Geometry: final body of the model. Coordinates: model frame, mm. Face numbers are marked on the shaded views. A direction names the side the tool comes from. Coordinates: 2 decimals unless noted, no trailing zeros. Write each loop counter-clockwise with the first axis right and the second up, starting at its lowest first coordinate (ties: lowest second). Pieces come first, ordered by that corner, then holes. Notation, with made-up numbers: (9, 46.5) -> (67, 46.5) arc R28 ccw to (67, 78.5) -> close; hole circle Ø6 at (0, 77). An arc over 180 degrees is marked (long way). One line per item, written item: value.
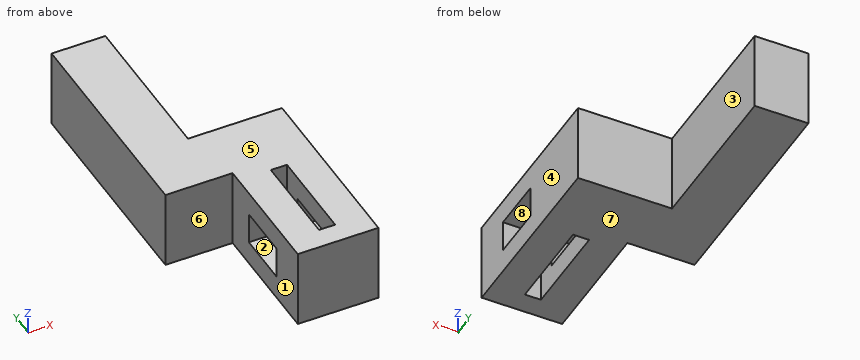
```python
from build123d import *

# Parameters (mm, degrees)
SKETCH1_W           = 30
SKETCH1_H           = 30
BOSS_EXTRUDE1_DEPTH = 70
SKETCH2_W           = 6
SKETCH2_H           = 35
CUT_EXTRUDE1_DEPTH  = 82.853527719
SKETCH3_W           = 12
SKETCH3_H           = 20
CUT_EXTRUDE2_DEPTH  = 82.853527719
SKETCH4_W           = 30
SKETCH4_H           = 22.669600449
BOSS_EXTRUDE2_DEPTH = 25
SKETCH5_W           = 20
SKETCH5_H           = 30
BOSS_EXTRUDE3_DEPTH = 60


with BuildPart() as part:
    # Sketch1 → Boss-Extrude1 (new body)
    with BuildSketch(Plane(origin=(0, 0, 0), x_dir=(1, 0, 0), z_dir=(0, 1, 0))):
        with Locations((15, -15)):
            Rectangle(SKETCH1_W, SKETCH1_H)
    extrude(amount=BOSS_EXTRUDE1_DEPTH)

    # Sketch2 → Cut-Extrude1 (cut, through all)
    with BuildSketch(Plane.XY.offset(30)):
        with Locations((15, 25.5)):
            Rectangle(SKETCH2_W, SKETCH2_H)
    extrude(amount=-CUT_EXTRUDE1_DEPTH, mode=Mode.SUBTRACT)

    # Sketch3 → Cut-Extrude2 (cut, through all)
    with BuildSketch(Plane(origin=(30, 0, 0), x_dir=(0, 0, -1), z_dir=(1, 0, 0))):
        with Locations((-15, 25.5)):
            Rectangle(SKETCH3_W, SKETCH3_H)
    extrude(amount=-CUT_EXTRUDE2_DEPTH, mode=Mode.SUBTRACT)

    # Sketch4 → Boss-Extrude2 (add)
    with BuildSketch(Plane.ZY):
        with Locations((15, 58.665199775)):
            Rectangle(SKETCH4_W, SKETCH4_H)
    extrude(amount=BOSS_EXTRUDE2_DEPTH)

    # Sketch5 → Boss-Extrude3 (add)
    with BuildSketch(Plane(origin=(0, 70, 0), x_dir=(1, 0, 0), z_dir=(0, 1, 0))):
        with Locations((-15, -15)):
            Rectangle(SKETCH5_W, SKETCH5_H)
    extrude(amount=BOSS_EXTRUDE3_DEPTH)


solid = part.part
```
(1) Reachability of the marked faces 1, 2, 3 and 4 from +Z, -Z, +X, -X, +Y, -Y: full face, straight path, thin tool, end or side. Return the list, or none.
Responses:
face 1: +Z, -Z, -X, -Y
face 2: +X, -X
face 3: +Z, -Z, +X, +Y
face 4: +Z, -Z, +X, +Y, -Y
(2) Section C-C (z = 15.25). Return the cut outline in (x, y).
Responses:
outline: (-25, 47.33) -> (0, 47.33) -> (0, 35.5) -> (12, 35.5) -> (12, 43) -> (18, 43) -> (18, 35.5) -> (30, 35.5) -> (30, 70) -> (-5, 70) -> (-5, 130) -> (-25, 130) -> close; (0, 0) -> (30, 0) -> (30, 15.5) -> (18, 15.5) -> (18, 8) -> (12, 8) -> (12, 15.5) -> (0, 15.5) -> close
(3) Section D-D (z = 28). Return the cut outline in (x, y), then the cut area to 3 significant figures.
Responses:
outline: (-25, 47.33) -> (0, 47.33) -> (0, 0) -> (30, 0) -> (30, 70) -> (-5, 70) -> (-5, 130) -> (-25, 130) -> close; hole (12, 8) -> (18, 8) -> (18, 43) -> (12, 43) -> close
area: 3,660 mm2
(4) Line query: line 1 (X direction, y = 34.5, z = 28); line 2 (Y direction, x = 14.5, z = 15); line 3 (Y direction, x = 18.5, z = 8.5). Output: solid intervals per line, ascending. Write a range as [from, to].
Responses:
line 1: x = [0, 12], [18, 30]
line 2: y = [0, 8], [43, 70]
line 3: y = [0, 70]
(5) Section A-A (y = 11.5). Return the cut outline in (x, z), then the cut area to 3 significant figures.
Responses:
outline: (0, 0) -> (12, 0) -> (12, 30) -> (0, 30) -> close; (18, 0) -> (30, 0) -> (30, 30) -> (18, 30) -> close
area: 720 mm2
(6) First-contact query: pin 1 (3.5 mm diameter, centred on x = 25, z = 16.5, fed in from -Y); pin 2 (3 mm diameter, centred on x = 8, z = 14, fed in from +Y); pin 3 (12.5 mm diameter, centred on x = -9, z = 21.5, fed in from -Y); pin 4 (15 mm diameter, centred on y = 18.5, z = 17.5, fed in from -X). Flat tips, straight axial feed; report the tip coordinate or a pass-through.
Responses:
pin 1: stops at y = 0
pin 2: stops at y = 70
pin 3: stops at y = 47.33
pin 4: stops at x = 0
(7) Section B-B (x = 7). Return the cut outline in (y, z), then the cut area to 3 significant figures.
Responses:
outline: (0, 0) -> (70, 0) -> (70, 30) -> (0, 30) -> close; hole (15.5, 9) -> (35.5, 9) -> (35.5, 21) -> (15.5, 21) -> close
area: 1,860 mm2
(8) Pull-direction query (Z, two-part tool) for the marked faces 5, 6, 7 and 8; classes: released by +Z, released by -Z, zero draft, split by the parting line, or undercut.
Responses:
face 5: released by +Z
face 6: zero draft
face 7: released by -Z
face 8: undercut
